```python
from build123d import *

# Parameters (mm, degrees)
PAD_DEPTH       = 75
SKETCH001_R     = 15
POCKET_DEPTH    = 3
SKETCH002_R     = 15
POCKET001_DEPTH = 3
SKETCH003_R     = 15
POCKET002_DEPTH = 3
SKETCH004_R     = 15
POCKET003_DEPTH = 3
SKETCH005_R     = 15
POCKET004_DEPTH = 3
SKETCH006_R     = 15
POCKET005_DEPTH = 3
SKETCH007_R     = 15
POCKET006_DEPTH = 3
SKETCH008_R     = 15
POCKET007_DEPTH = 3
SKETCH009_R     = 15
POCKET008_DEPTH = 3
SKETCH010_R     = 15
POCKET009_DEPTH = 3
SKETCH011_R     = 15
POCKET010_DEPTH = 3
SKETCH012_R     = 15
POCKET011_DEPTH = 3
SKETCH013_W     = 16.6623057169
SKETCH013_H     = 10
PAD001_DEPTH    = 12
SKETCH014_W     = 16.6623057169
SKETCH014_H     = 10
PAD002_DEPTH    = 12
SKETCH015_W     = 16.6623057169
SKETCH015_H     = 10
PAD003_DEPTH    = 12
SKETCH016_W     = 16.6623057169
SKETCH016_H     = 10
PAD004_DEPTH    = 12
SKETCH017_W     = 16.6623057169
SKETCH017_H     = 10
PAD005_DEPTH    = 12
SKETCH018_R     = 2
PAD006_DEPTH    = 3
SKETCH019_R     = 2
PAD007_DEPTH    = 3
SKETCH020_R     = 2
PAD008_DEPTH    = 3
SKETCH021_R     = 2
PAD009_DEPTH    = 3


with BuildPart() as part:
    # Sketch → Pad (new body)
    with BuildSketch(Plane.XZ):
        Polygon((-115, 15), (-115, -15), (-109.3011558106, -30.6574457275), (-90.01752752, -53.638779021), (-75.5875474835, -61.9699318795), (-46.6097726948, -69.7345032326), (-15, -72.5), (15, -72.5), (46.6097726948, -69.7345032326), (75.5875474835, -61.9699318795), (90.01752752, -53.638779021), (109.3011558106, -30.6574457275), (115, -15), (115, 15), (109.3011558106, 30.6574457275), (90.01752752, 53.638779021), (75.5875474835, 61.9699318795), (46.6097726948, 69.7345032326), (15, 72.5), (-15, 72.5), (-46.6097726948, 69.7345032326), (-75.5875474835, 61.9699318795), (-90.01752752, 53.638779021), (-109.3011558106, 30.6574457275), align=None)
        Polygon((-15, 70.5), (15, 70.5), (45.1474724059, 67.8624379305), (73.5017505011, 60.2649320129), (87.4928960516, 52.1871403631), (107.1664449714, 28.7411177589), (112.4249806172, 14.2934098125), (112.4249806172, -15.129325967), (107.2690057988, -29.295250356), (87.1410348375, -53.2828320607), (75.2862851494, -60.1271749843), (46.7496758605, -67.773536398), (15.5584899901, -70.5024115636), (-14.9018142644, -70.5024115636), (-45.3108694437, -67.8419639668), (-73.8953035194, -60.1827879401), (-87.3182795517, -52.4330291146), (-106.7555862722, -29.268549), (-112.8239045631, -15.209551), (-112.8239045631, 14.0555263106), (-107.3779577019, 29.0181423395), (-87.4996413362, 52.708197283), (-74.455381738, 60.2393040734), (-46.4214173604, 67.7509821891), align=None, mode=Mode.SUBTRACT)
    extrude(amount=PAD_DEPTH)

    # Sketch001 (on Face24 of Pad) → Pocket (cut)
    with BuildSketch(Plane(origin=(0, 0, 72.5), x_dir=(-1, 0, 0), z_dir=(0, 0, 1))):
        with Locations((0, 37.5)):
            Circle(SKETCH001_R)
    extrude(amount=-POCKET_DEPTH, mode=Mode.SUBTRACT)

    # Sketch002 (on Face28 of Pocket) → Pocket001 (cut)
    with BuildSketch(Plane(origin=(20.5558885464, 0, 76.7156204498), x_dir=(-0.9659258263, 0, 0.2588190451), z_dir=(0.2588190451, 0, 0.9659258263))):
        with Locations((-41.972965666, 37.5)):
            Circle(SKETCH002_R)
    extrude(amount=-POCKET001_DEPTH, mode=Mode.SUBTRACT)

    # Sketch003 (on Face4 of Pocket001) → Pocket002 (cut)
    with BuildSketch(Plane(origin=(-20.5558885464, 0, 76.7156204498), x_dir=(-0.9659258263, 0, -0.2588190451), z_dir=(-0.2588190451, 0, 0.9659258263))):
        with Locations((41.972965666, 37.5)):
            Circle(SKETCH003_R)
    extrude(amount=-POCKET002_DEPTH, mode=Mode.SUBTRACT)

    # Sketch004 (on Face28 of Pocket002) → Pocket003 (cut)
    with BuildSketch(Plane(origin=(79.236396287, 0, 66.4872309002), x_dir=(-0.6427876097, 0, 0.7660444431), z_dir=(0.7660444431, 0, 0.6427876097))):
        with Locations((-31.7724627397, 37.5)):
            Circle(SKETCH004_R)
    extrude(amount=-POCKET003_DEPTH, mode=Mode.SUBTRACT)

    # Sketch005 (on Face12 of Pocket003) → Pocket004 (cut)
    with BuildSketch(Plane(origin=(-79.236396287, 0, 66.4872309002), x_dir=(-0.6427876097, 0, -0.7660444431), z_dir=(-0.7660444431, 0, 0.6427876097))):
        with Locations((31.7724627397, 37.5)):
            Circle(SKETCH005_R)
    extrude(amount=-POCKET004_DEPTH, mode=Mode.SUBTRACT)

    # Sketch006 (on Face26 of Pocket004) → Pocket005 (cut)
    with BuildSketch(Plane(origin=(115, 0, 0), x_dir=(0, 0, 1), z_dir=(1, 0, 0))):
        with Locations((0, 37.5)):
            Circle(SKETCH006_R)
    extrude(amount=-POCKET005_DEPTH, mode=Mode.SUBTRACT)

    # Sketch007 (on Face14 of Pocket005) → Pocket006 (cut)
    with BuildSketch(Plane(origin=(-115, 0, 0), x_dir=(0, 0, -1), z_dir=(-1, 0, 0))):
        with Locations((0, 37.5)):
            Circle(SKETCH007_R)
    extrude(amount=-POCKET006_DEPTH, mode=Mode.SUBTRACT)

    # Sketch008 (on Face16 of Pocket006) → Pocket007 (cut)
    with BuildSketch(Plane(origin=(-79.236396287, 0, -66.4872309002), x_dir=(0.6427876097, 0, -0.7660444431), z_dir=(-0.7660444431, 0, -0.6427876097))):
        with Locations((-31.7724627397, 37.5)):
            Circle(SKETCH008_R)
    extrude(amount=-POCKET007_DEPTH, mode=Mode.SUBTRACT)

    # Sketch009 (on Face18 of Pocket007) → Pocket008 (cut)
    with BuildSketch(Plane(origin=(-20.5558885464, 0, -76.7156204498), x_dir=(0.9659258263, 0, -0.2588190451), z_dir=(-0.2588190451, 0, -0.9659258263))):
        with Locations((-41.972965666, 37.5)):
            Circle(SKETCH009_R)
    extrude(amount=-POCKET008_DEPTH, mode=Mode.SUBTRACT)

    # Sketch010 (on Face20 of Pocket008) → Pocket009 (cut)
    with BuildSketch(Plane(origin=(0, 0, -72.5), x_dir=(1, 0, 0), z_dir=(0, 0, -1))):
        with Locations((0, 37.5)):
            Circle(SKETCH010_R)
    extrude(amount=-POCKET009_DEPTH, mode=Mode.SUBTRACT)

    # Sketch011 (on Face22 of Pocket009) → Pocket010 (cut)
    with BuildSketch(Plane(origin=(20.5558885464, 0, -76.7156204498), x_dir=(0.9659258263, 0, 0.2588190451), z_dir=(0.2588190451, 0, -0.9659258263))):
        with Locations((41.972965666, 37.5)):
            Circle(SKETCH011_R)
    extrude(amount=-POCKET010_DEPTH, mode=Mode.SUBTRACT)

    # Sketch012 (on Face24 of Pocket010) → Pocket011 (cut)
    with BuildSketch(Plane(origin=(79.236396287, 0, -66.4872309002), x_dir=(0.6427876097, 0, 0.7660444431), z_dir=(0.7660444431, 0, -0.6427876097))):
        with Locations((31.7724627397, 37.5)):
            Circle(SKETCH012_R)
    extrude(amount=-POCKET011_DEPTH, mode=Mode.SUBTRACT)

    # Sketch013 (on Face29 of Pocket011) → Pad001 (join)
    with BuildSketch(Plane(origin=(45.7306545101, 0, 79.2078170749), x_dir=(-0.8660254038, 0, 0.5), z_dir=(0.5, 0, 0.8660254038))):
        with Locations((-42.8069232492, 10)):
            Rectangle(SKETCH013_W, SKETCH013_H)
        with Locations((-42.8069232492, 70)):
            Rectangle(SKETCH013_W, SKETCH013_H)
    extrude(amount=PAD001_DEPTH)

    # Sketch014 (on Face10 of Pad001) → Pad002 (join)
    with BuildSketch(Plane(origin=(-45.7306545101, 0, 79.2078170749), x_dir=(-0.8660254038, 0, -0.5), z_dir=(-0.5, 0, 0.8660254038))):
        with Locations((42.8069232492, 10)):
            Rectangle(SKETCH014_W, SKETCH014_H)
    extrude(amount=PAD002_DEPTH)

    # Sketch015 (on Face19 of Pad002) → Pad003 (join)
    with BuildSketch(Plane(origin=(-45.7306545101, 0, -79.2078170749), x_dir=(0.8660254038, 0, -0.5), z_dir=(-0.5, 0, -0.8660254038))):
        with Locations((-42.8069232492, 10)):
            Rectangle(SKETCH015_W, SKETCH015_H)
        with Locations((-42.8069232492, 70)):
            Rectangle(SKETCH015_W, SKETCH015_H)
    extrude(amount=PAD003_DEPTH)

    # Sketch016 (on Face25 of Pad003) → Pad004 (join)
    with BuildSketch(Plane(origin=(45.7306545101, 0, -79.2078170749), x_dir=(0.8660254038, 0, 0.5), z_dir=(0.5, 0, -0.8660254038))):
        with Locations((42.8069232492, 10)):
            Rectangle(SKETCH016_W, SKETCH016_H)
        with Locations((42.8069232492, 70)):
            Rectangle(SKETCH016_W, SKETCH016_H)
    extrude(amount=PAD004_DEPTH)

    # Sketch017 (on Face12 of Pad004) → Pad005 (join)
    with BuildSketch(Plane(origin=(-45.7306545101, 0, 79.2078170749), x_dir=(-0.8660254038, 0, -0.5), z_dir=(-0.5, 0, 0.8660254038))):
        with Locations((42.8069232492, 70)):
            Rectangle(SKETCH017_W, SKETCH017_H)
    extrude(amount=PAD005_DEPTH)

    # Sketch018 (on Face1 of Pad005) → Pad006 (join)
    with BuildSketch(Plane(origin=(-6.4086882928, 0, 73.2516423792), x_dir=(-0.9961946981, 0, -0.0871557427), z_dir=(-0.0871557427, 0, 0.9961946981))):
        with Locations((30.3241291222, 61)):
            Circle(SKETCH018_R)
        with Locations((18.9241291222, 61)):
            Circle(SKETCH018_R)
        with Locations((18.9241291222, 14)):
            Circle(SKETCH018_R)
        with Locations((30.3241291222, 14)):
            Circle(SKETCH018_R)
    extrude(amount=PAD006_DEPTH)

    # Sketch019 (on Face12 of Pad006) → Pad007 (join)
    with BuildSketch(Plane(origin=(6.4086882928, 0, 73.2516423792), x_dir=(-0.9961946981, 0, 0.0871557427), z_dir=(0.0871557427, 0, 0.9961946981))):
        with Locations((-30.0546460135, 61)):
            Circle(SKETCH019_R)
        with Locations((-18.6546460135, 61)):
            Circle(SKETCH019_R)
        with Locations((-18.6546460135, 14)):
            Circle(SKETCH019_R)
        with Locations((-30.0546460135, 14)):
            Circle(SKETCH019_R)
    extrude(amount=PAD007_DEPTH)

    # Sketch020 (on Face22 of Pad007) → Pad008 (join)
    with BuildSketch(Plane(origin=(-6.4086882928, 0, -73.2516423792), x_dir=(0.9961946981, 0, -0.0871557427), z_dir=(-0.0871557427, 0, -0.9961946981))):
        with Locations((-30.0546460135, 61)):
            Circle(SKETCH020_R)
        with Locations((-18.6546460135, 61)):
            Circle(SKETCH020_R)
        with Locations((-30.0546460135, 14)):
            Circle(SKETCH020_R)
        with Locations((-18.6546460135, 14)):
            Circle(SKETCH020_R)
    extrude(amount=PAD008_DEPTH)

    # Sketch021 (on Face24 of Pad008) → Pad009 (join)
    with BuildSketch(Plane(origin=(6.4086882928, 0, -73.2516423792), x_dir=(0.9961946981, 0, 0.0871557427), z_dir=(0.0871557427, 0, -0.9961946981))):
        with Locations((18.9241291222, 61)):
            Circle(SKETCH021_R)
        with Locations((30.3241291222, 61)):
            Circle(SKETCH021_R)
        with Locations((18.9241291222, 14)):
            Circle(SKETCH021_R)
        with Locations((30.3241291222, 14)):
            Circle(SKETCH021_R)
    extrude(amount=PAD009_DEPTH)


solid = part.part
```
Part model, mm, in its own coordinate system. A direction names the side the tool comes from. Coordinates: 2 decimals unless noted, no trailing zeros. Loops run counter-clockwise (first coordinate to the right, second up) from the corner with the lowest first, then second, coordinate; pieces in that order, holes last. Notation, with made-up numbers: (18, 36.5) - (76, 36.5) arc R21 ccw to (76, 41.5) - close; hole circle Ø7 at (6.25, 14). An arc over 180 degrees is marked (long way). Write item = value, one per line. Start each with the question number.
Item 1: Cut at A-A, the plane x = 0. Give the cut face in (y, z), and give its area (3 significant figures).
Item 2: Cut at C-C, the plane z = 17.5. Give the cut face in (x, y), and give its area (3 significant figures).
Item 3: Mould opens along X. For faces 6 (the flat face through (-88.9, -10.07, -68.14)), 7 (the flat face through (-86, -65, -63)), 8 (the flat face through (30.584, -36.975, -71.137)), 9 (the flat face through (92.976, -9.93, 58.762)) say: released by +X, released by -X, zero draft, split by the parting line, or undercut.
Item 4: Cut at B-B, the plane z = -1.5. Give the cut face in (x, y).
Item 5: 3-axis set-ups, long thin cutter, end or side, ignore diameter. For faces 1 (the flat face through (-92.976, -9.93, -58.762)), 2 (the flat face through (-78.546, -9.93, 67.093)), 3 (the flat face through (86, -5, 63)), 4 (the flat face through (0, -64, -72.5)), 5 (the flat face through (46.5, -28.6, 67.5)): which of +Z, -Z, +X, -X, +Y, -Y reach the whole face in a straight line?
Item 6: Wall check: L1, parallel to Z at x = 3.5, y = -66; L2, parallel to X at y = -70.5, z = -14; L3, parallel to Y at x = 0, z = -71.6. Give the ranges that are in metal, low to high. Write a range as from..to.
Item 7: Flat gauge pins, fed straight in: pin 1 Ø15 at (x, y) = (5.5, -51) entering from +Z; pin 2 Ø1 at (x, y) = (-86.5, -18.5) entering from +Z; pin 3 Ø24 at (x, y) = (2, -62) entering from -Z. Where does each tip first touch, or does it go through?
The answers:
q1.outline = (-75, -72.5) - (-52.5, -72.5) - (-52.5, -70.5) - (-75, -70.5) - close; (-75, 70.5) - (-52.5, 70.5) - (-52.5, 72.5) - (-75, 72.5) - close; (-22.5, -72.5) - (0, -72.5) - (0, -70.5) - (-22.5, -70.5) - close; (-22.5, 70.5) - (0, 70.5) - (0, 72.5) - (-22.5, 72.5) - close
q1.area = 180 mm2
q2.outline = (-114.09, -75) - (-111.57, -75) - (-111.57, 0) - (-114.09, 0) - close; (111.26, -75) - (114.09, -75) - (114.09, 0) - (111.26, 0) - close
q2.area = 401 mm2
q3.face_6 = released by -X
q3.face_7 = zero draft
q3.face_8 = undercut
q3.face_9 = released by +X
q4.outline = (-115, -75) - (-112.82, -75) - (-112.82, -52.42) - (-115, -52.42) - close; (-115, -22.58) - (-112.82, -22.58) - (-112.82, 0) - (-115, 0) - close; (112.42, -75) - (115, -75) - (115, -52.42) - (112.42, -52.42) - close; (112.42, -22.58) - (115, -22.58) - (115, 0) - (112.42, 0) - close
q5.face_1 = -X, +Y, -Y
q5.face_2 = +Z, +Y, -Y
q5.face_3 = +Z, +X, +Y
q5.face_4 = -Z, +Y, -Y
q5.face_5 = +Y, -Y
q6.L1 = -72.5..-70.5, 70.5..72.5
q6.L2 = -115..-112.82, 112.42..115
q6.L3 = -75..-52.5, -22.5..0
q7.pin_1 = 72.5
q7.pin_2 = 55.96
q7.pin_3 = -72.5
